Geometry: final body of the model. Coordinates: model frame, mm. A direction names the side the tool comes from. Give positions to 0.01 mm unless a question says otherwise; leave off trailing zeros. Order: outer loops, then holes, each group sorted by start corner. A loop starts at its lowest first (then second) coordinate and runs counter-clockwise, first axis right, second up. Notation, with made-up numbers: (68, 72) -> (98, 72) arc R23 ccw to (98, 84) -> close; hole circle Ø11 at (-11.5, -31). An arc over 180 degrees is marked (long way). One line per question, with ' | ' between items.
from build123d import *

# Parameters (mm, degrees)
F0_W          = 74.4
F0_H          = 39.1
F0_R          = 1
F0_R_2        = 4.1
F1_DEPTH      = 1.5
F2_W          = 74.4
F2_H          = 35
F3_DEPTH      = 1.5
F4_W          = 25.6
F4_H          = 24.2
F5_DEPTH      = 1.5
F6_R          = 10
F7_W          = 1.5
F7_H          = 37
F8_DEPTH      = 24
F8_DEPTH_BACK = 1.5
F9_R          = 1.1
F9_R_2        = 4.05
F10_DEPTH     = 1.5


with BuildPart() as f1:
    # F0 (on Top) → F1 (new body)
    with BuildSketch(Plane.XY):
        Rectangle(F0_W, F0_H)
        with Locations((-32.2, -16.55)):
            Circle(F0_R, mode=Mode.SUBTRACT)
        with Locations((-25, -10.35)):
            Circle(F0_R_2, mode=Mode.SUBTRACT)
        with Locations((-17.8, -16.55)):
            Circle(F0_R, mode=Mode.SUBTRACT)
        with Locations((17.8, -16.55)):
            Circle(F0_R, mode=Mode.SUBTRACT)
        with Locations((32.2, -16.55)):
            Circle(F0_R, mode=Mode.SUBTRACT)
        with Locations((25, -10.35)):
            Circle(F0_R_2, mode=Mode.SUBTRACT)
        with BuildLine():
            ThreePointArc((-34.8, 11.35), (-34.507107, 12.057107), (-33.8, 12.35))
            Line((-33.8, 12.35), (-30.123475, 12.35))
            ThreePointArc((-30.123475, 12.35), (-25, 14.85), (-19.876525, 12.35))
            Line((-19.876525, 12.35), (-16.2, 12.35))
            ThreePointArc((-16.2, 12.35), (-15.492893, 12.057107), (-15.2, 11.35))
            Line((-15.2, 11.35), (-15.2, 1.65))
            ThreePointArc((-15.2, 1.65), (-16.664466, -1.885534), (-20.2, -3.35))
            Line((-20.2, -3.35), (-29.8, -3.35))
            ThreePointArc((-29.8, -3.35), (-33.335534, -1.885534), (-34.8, 1.65))
            Line((-34.8, 1.65), (-34.8, 11.35))
        make_face(mode=Mode.SUBTRACT)
        with Locations((-32.7, 14.55)):
            Circle(F0_R, mode=Mode.SUBTRACT)
        with Locations((-17.3, 14.55)):
            Circle(F0_R, mode=Mode.SUBTRACT)
        with BuildLine():
            Line((15.2, 1.65), (15.2, 11.35))
            ThreePointArc((15.2, 11.35), (15.492893, 12.057107), (16.2, 12.35))
            Line((16.2, 12.35), (19.876525, 12.35))
            ThreePointArc((19.876525, 12.35), (25, 14.85), (30.123475, 12.35))
            Line((30.123475, 12.35), (33.8, 12.35))
            ThreePointArc((33.8, 12.35), (34.507107, 12.057107), (34.8, 11.35))
            Line((34.8, 11.35), (34.8, 1.65))
            ThreePointArc((34.8, 1.65), (33.335534, -1.885534), (29.8, -3.35))
            Line((29.8, -3.35), (20.2, -3.35))
            ThreePointArc((20.2, -3.35), (16.664466, -1.885534), (15.2, 1.65))
        make_face(mode=Mode.SUBTRACT)
        with Locations((17.3, 14.55)):
            Circle(F0_R, mode=Mode.SUBTRACT)
        with Locations((32.7, 14.55)):
            Circle(F0_R, mode=Mode.SUBTRACT)
    extrude(amount=F1_DEPTH)

    # F2 (on face) → F3 (join)
    with BuildSketch(Plane.XY.offset(1.5)):
        with Locations((0, 37.05)):
            Rectangle(F2_W, F2_H)
    extrude(amount=-F3_DEPTH)

    # F4 (on face) → F5 (cut, through all)
    with BuildSketch(Plane.XY.offset(1.5)):
        with Locations((0, -7.45)):
            Rectangle(F4_W, F4_H)
    extrude(amount=-F5_DEPTH, mode=Mode.SUBTRACT)

    # F6
    f6_edges = [f1.edges().sort_by_distance(p)[0] for p in [
        (-12.8, 4.65, 0.75),
        (12.8, 4.65, 0.75),
    ]]
    fillet(f6_edges, radius=F6_R)

    # F7 (on face) → F8 (join, two sides)
    with BuildSketch(Plane.XY.offset(1.5)) as f8_sk:
        with Locations((37.95, 36.05)):
            Rectangle(F7_W, F7_H)
    extrude(amount=F8_DEPTH)
    extrude(f8_sk.sketch, amount=-F8_DEPTH_BACK)

    # F9 (on face) → F10 (cut, through all)
    with BuildSketch(Plane.YZ.offset(38.7)):
        with Locations((51.6, 20.7)):
            Circle(F9_R)
        with Locations((45.4, 13.5)):
            Circle(F9_R_2)
        with BuildLine():
            ThreePointArc((38.4, 18.3), (36.935534, 21.835534), (33.4, 23.3))
            Line((33.4, 23.3), (22.7, 23.3))
            Line((22.7, 23.3), (22.7, 3.7))
            Line((22.7, 3.7), (33.4, 3.7))
            ThreePointArc((33.4, 3.7), (36.935534, 5.164466), (38.4, 8.7))
            Line((38.4, 8.7), (38.4, 18.3))
        make_face()
        with Locations((51.6, 6.3)):
            Circle(F9_R)
        with Locations((20.5, 21.2)):
            Circle(F9_R)
        with Locations((20.5, 5.8)):
            Circle(F9_R)
    extrude(amount=-F10_DEPTH, mode=Mode.SUBTRACT)

    # F11: F1 across plane


with BuildPart() as f1_1:
    add(f1.part)
    add(f1.part.mirror(Plane.YZ))


solid = f1_1.part
1) Section A-A on y = 31.5. Return loops of the section in (x, z).
Check result:
outline: (-38.7, 0) -> (38.7, 0) -> (38.7, 3.7) -> (37.2, 3.7) -> (37.2, 1.5) -> (-37.2, 1.5) -> (-37.2, 3.7) -> (-38.7, 3.7) -> close; (-38.7, 23.3) -> (-37.2, 23.3) -> (-37.2, 25.5) -> (-38.7, 25.5) -> close; (37.2, 23.3) -> (38.7, 23.3) -> (38.7, 25.5) -> (37.2, 25.5) -> close
2) Section C-C on z = 10.5. Return loops of the section in (x, y), plus the area to 3 significant figures.
Check result:
outline: (-38.7, 17.55) -> (-37.2, 17.55) -> (-37.2, 22.7) -> (-38.7, 22.7) -> close; (-38.7, 38.4) -> (-37.2, 38.4) -> (-37.2, 42.68) -> (-38.7, 42.68) -> close; (-38.7, 48.12) -> (-37.2, 48.12) -> (-37.2, 54.55) -> (-38.7, 54.55) -> close; (37.2, 17.55) -> (38.7, 17.55) -> (38.7, 22.7) -> (37.2, 22.7) -> close; (37.2, 38.4) -> (38.7, 38.4) -> (38.7, 42.68) -> (37.2, 42.68) -> close; (37.2, 48.12) -> (38.7, 48.12) -> (38.7, 54.55) -> (37.2, 54.55) -> close | area: 47.6 mm^2
3) Contact query for flat-ended pins moving along their axis: pin 1 Ø5 at (x, z) = (-10.5, 6) entering from -Y; pin 2 Ø4 at (x, y) = (25, 26) entering from +Z; pin 3 Ø1.6 at (x, z) = (-38, 12.5) entering from -Y; pin 4 Ø1.2 at (y, z) = (4.5, 0.5) entering from +X. Output: stop coordinate, or through.
Check result:
pin 1: passes through | pin 2: stops at z = 1.5 | pin 3: stops at y = 17.55 | pin 4: stops at x = 37.2
4) Section B-B on x = 25. Return loops of the section in (y, z).
Check result:
outline: (-19.55, 0) -> (-14.45, 0) -> (-14.45, 1.5) -> (-19.55, 1.5) -> close; (-6.25, 0) -> (-3.35, 0) -> (-3.35, 1.5) -> (-6.25, 1.5) -> close; (14.85, 0) -> (54.55, 0) -> (54.55, 1.5) -> (14.85, 1.5) -> close
5) Section D-D on y = 45.4. Return loops of the section in (x, z).
Check result:
outline: (-38.7, 0) -> (38.7, 0) -> (38.7, 9.45) -> (37.2, 9.45) -> (37.2, 1.5) -> (-37.2, 1.5) -> (-37.2, 9.45) -> (-38.7, 9.45) -> close; (-38.7, 17.55) -> (-37.2, 17.55) -> (-37.2, 25.5) -> (-38.7, 25.5) -> close; (37.2, 17.55) -> (38.7, 17.55) -> (38.7, 25.5) -> (37.2, 25.5) -> close
6) Material intervals for probe 1 along Z at (x, y) = (37.6, 20.5); probe 2 along X at (y, z) = (-10.35, 1.25); probe 3 along X at (y, z) = (47, 22.5), sorted ascending. Write a range as from..to.
Check result:
probe 1: z = 0..4.7, 6.9..20.1, 22.3..25.5 | probe 2: x = -37.2..-29.1, -20.9..-12.8, 12.8..20.9, 29.1..37.2 | probe 3: x = -38.7..-37.2, 37.2..38.7
7) Pull-direction query (Z, two-part tool) for faces 1 (the cylindrical face through (37.96, 36.9, 5.13)), 2 (the flat face through (1, 26, 0)), 3 (the flat face through (-1, 26, 1.5)); classes: +Z half, -Z half, draft (parallel to the pull), parting line (faces both ways), or undercut.
Check result:
face 1: undercut | face 2: -Z half | face 3: +Z half
8) Set-up query: faces 4 (the cylindrical face through (-16.63, -1.85, 0.74)), 5 (the cylindrical face through (-38, 50.5, 20.7)), 6 (the cylindrical face through (9.95, 1.64, 0.74)). Return all of +Z, -Z, +X, -X, +Y, -Y with unobstructed straight access to the full face (end or side cutting, diameter ignored); none if empty.
Check result:
face 4: +Z, -Z | face 5: +X, -X | face 6: +Z, -Z, -Y
